```python
from build123d import *

# Parameters (mm, degrees)
SKETCH1_W           = 21
SKETCH1_H           = 5
BOSS_EXTRUDE1_DEPTH = 5
SKETCH2_W           = 10
SKETCH2_H           = 16
BOSS_EXTRUDE2_DEPTH = 12.8
SKETCH3_R           = 1.25
CUT_EXTRUDE1_DEPTH  = 13
SKETCH4_R           = 5
CUT_EXTRUDE2_DEPTH  = 13


with BuildPart() as part:
    # Sketch1 → Boss-Extrude1 (new body)
    with BuildSketch(Plane.XY):
        with Locations((10.5, 2.5)):
            Rectangle(SKETCH1_W, SKETCH1_H)
    extrude(amount=BOSS_EXTRUDE1_DEPTH)

    # Sketch2 → Boss-Extrude2 (add)
    with BuildSketch(Plane(origin=(0, 5, 0), x_dir=(1, 0, 0), z_dir=(0, 1, 0))):
        with Locations((10.5, 3)):
            Rectangle(SKETCH2_W, SKETCH2_H)
    extrude(amount=BOSS_EXTRUDE2_DEPTH)

    # Sketch3 → Cut-Extrude1 (cut)
    with BuildSketch(Plane(origin=(0, 5, 0), x_dir=(1, 0, 0), z_dir=(0, 1, 0))):
        with Locations(Location((3, -2.5, 0), (0, 0, 270))):
            Circle(SKETCH3_R)
        with Locations(Location((18, -2.5, 0), (0, 0, 270))):
            Circle(SKETCH3_R)
    extrude(amount=-CUT_EXTRUDE1_DEPTH, mode=Mode.SUBTRACT)

    # Sketch4 → Cut-Extrude2 (cut)
    with BuildSketch(Plane(origin=(15.5, 0, 0), x_dir=(0, 0, -1), z_dir=(1, 0, 0))):
        with Locations((5.5, 11.4)):
            Circle(SKETCH4_R)
    extrude(amount=-CUT_EXTRUDE2_DEPTH, mode=Mode.SUBTRACT)


solid = part.part
```
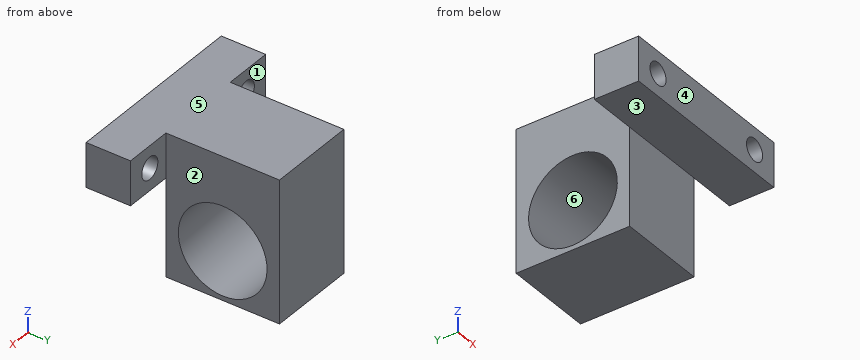
Could you check a few things on this model? Use its own coordinates, in mm. Face numbers are marked on the shaded views. A direction names the side the tool comes from. Give positions to 0.01 mm unless a question says otherwise; leave off trailing zeros. Loops run counter-clockwise (first coordinate to the right, second up) from the corner with the lowest first, then second, coordinate; pieces in that order, holes last. Notation, with made-up numbers: (60.5, 64.25) - (79.5, 64.25) arc R23 cw to (79.5, 82.25) - close; hole circle Ø11 at (52, 16). An arc over 180 degrees is marked (long way). Answer in a Markdown table with one row per item. Add a question column.
Q1. If we section it at C-C (x = 11.75): List the corners of the cut face in (y, z) for me.
Q2. We'd pull the mould along Z, two halves only. Please class the marked faces 4, 5 and 6: +Z half, -Z half, draft (parallel to the pull), parting line (faces both ways), or undercut.
Q3. If we section it at A-A (z = -5.5): List the corners of the cut face in (x, y) for me.
Q4. If we section it at D-D (z = 2.5): List the corners of the cut face in (x, y) for me.
Q5. If we section it at B-B (y = 11.4): List the corners of the cut face in (x, z) for me.
Q6. For pin 1 (2 mm diameter, centred on x = 8, y = 2.5, fed in from -Z); pin 2 (5 mm diameter, centred on x = 11, z = -8, fed in from -Y); pin 3 (2 mm diameter, centred on y = 15, z = 1, fed in from +X); pin 4 (1.5 mm diameter, centred on x = 18, z = 2.5, fed in from -Y), each with a flat end and sliding along its axis, tell me the tip position at first contact or that it passes through.
Q7. Please list where these lines run through material, in increasing order: L1, parallel to X at y = 1.6, z = 2.5; L2, parallel to Y at x = 8, z = -5.75; L3, parallel to Y at x = 4.5, z = 3.25. Write a range as from..to.
Q8. Which directions (+Z, -Z, +X, -X, +Y, -Y) give clear straight access to the entire face, cutting with the end or side of a thin tool? Please do the marked faces 1, 2 and 3.
The answers:
| question | item | result |
|---|---|---|
| 1 | outline | (0, 0) - (5, 0) - (5, -11) - (17.8, -11) - (17.8, 5) - (0, 5) - close; hole circle Ø10 at (11.4, -5.5) |
| 2 | face 4 | draft |
| 2 | face 5 | +Z half |
| 2 | face 6 | undercut |
| 3 | outline | (5.5, 5) - (15.5, 5) - (15.5, 6.4) - (5.5, 6.4) - close; (5.5, 16.4) - (15.5, 16.4) - (15.5, 17.8) - (5.5, 17.8) - close |
| 4 | outline | (0, 0) - (1.75, 0) - (1.75, 5) - (0, 5) - close; (4.25, 0) - (16.75, 0) - (16.75, 5) - (15.5, 5) - (15.5, 17.8) - (5.5, 17.8) - (5.5, 5) - (4.25, 5) - close; (19.25, 0) - (21, 0) - (21, 5) - (19.25, 5) - close |
| 5 | outline | (5.5, -11) - (15.5, -11) - (15.5, -10.5) - (5.5, -10.5) - close; (5.5, -0.5) - (15.5, -0.5) - (15.5, 5) - (5.5, 5) - close |
| 6 | pin 1 | stops at z = 0 |
| 6 | pin 2 | stops at y = 5 |
| 6 | pin 3 | stops at x = 15.5 |
| 6 | pin 4 | passes through |
| 7 | L1 | x = 0..1.75, 4.25..16.75, 19.25..21 |
| 7 | L2 | y = 5..6.41, 16.39..17.8 |
| 7 | L3 | y = 0..5 |
| 8 | face 1 | +Z, -Z, -X, +Y |
| 8 | face 2 | +Z, -Z, +X, +Y |
| 8 | face 3 | -Z, +X, -X, -Y |
